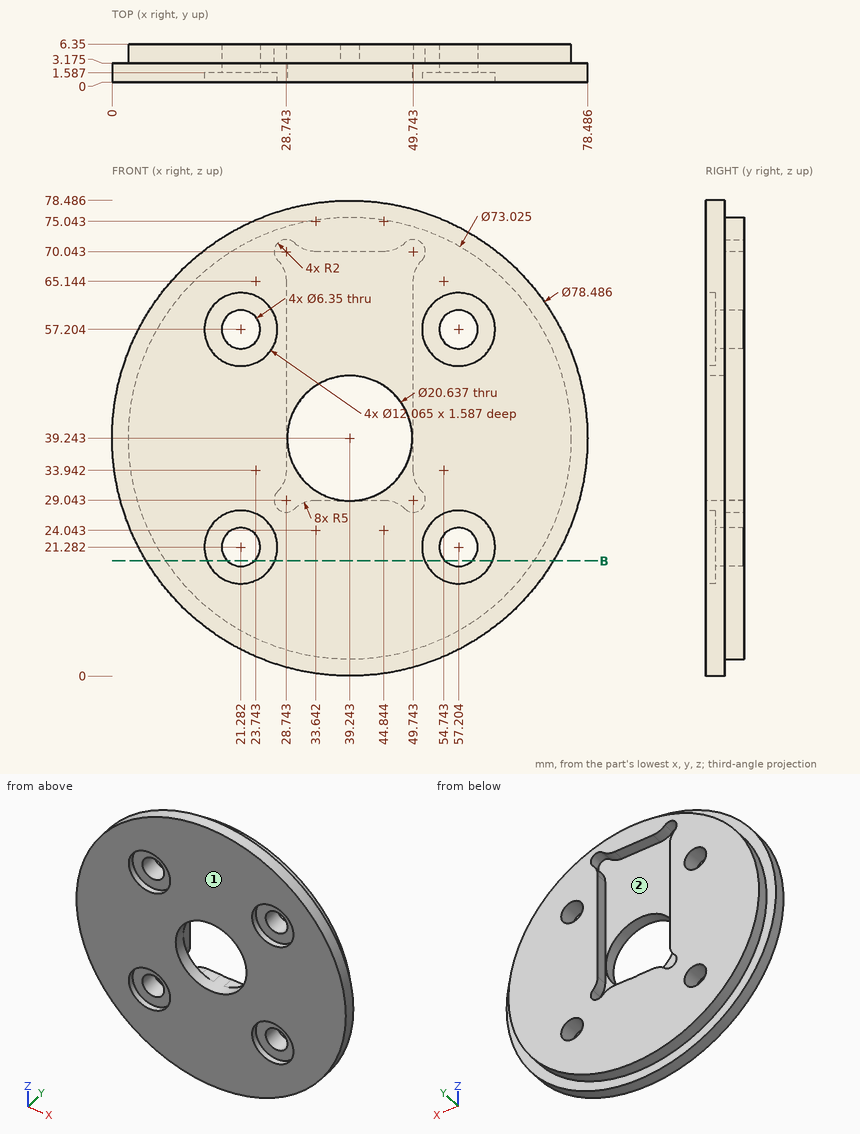
Verification items for this drawing (mm, ordinates from the low corner). Round coordinates to 2 decimals unless told otherwise and drop trailing zeros. Answer in a Markdown table with one row per item. Add a question column.
Item 1: Sectioned sample at B-B, the plane z = 19. State how many separate pieces and enclosed holes the cut face has, plus the area to 3 significant figures.
Item 2: Draft check along X on the marked faces 1 and 2. Enter one of: released by +X, released by -X, zero draft, split by the parting line, or undercut.
Item 3: Material ranges on L1, parallel to Z at x = 58, y = 5.75 (1 decimal); L2, parallel to Z at x = 19.5, y = 3.25 (1 decimal); L3, parallel to X at y = 6, z = 55 (1 decimal), recorded low to high. Write a range as [from, to].
Item 4: Depth check by flat-ended pin: pin 1 Ø3 at (y, z) = (3.5, 48) entering from -X; pin 2 Ø1.5 at (x, y) = (15, 1.5) entering from -Z; pin 3 Ø1 at (y, z) = (4, 50.5) entering from +X (1 decimal). Enter the tip coordinate at first touch or a pass-through.
Filled in:
| question | item | result |
|---|---|---|
| 1 | separate pieces | 3 |
| 1 | enclosed holes | 0 |
| 1 | area | 329 mm² |
| 2 | face 1 | zero draft |
| 2 | face 2 | undercut |
| 3 | L1 | z = [7.9, 18.2], [24.4, 54.1], [60.3, 70.6] |
| 3 | L2 | z = [8.5, 18.7], [23.9, 54.6], [59.8, 70] |
| 3 | L3 | x = [6.3, 19], [23.6, 28.7], [49.7, 54.9], [59.5, 72.2] |
| 4 | pin 1 | stops at x = 0.68 |
| 4 | pin 2 | stops at z = 7.81 |
| 4 | pin 3 | stops at x = 74.1 |
